Verification items for the finished model (mm, model axes). Round coordinates to 2 decimals unless told otherwise and drop trailing zeros. Write each loop counter-clockwise with the first axis right and the second up, starting at its lowest first coordinate (ties: lowest second). Pieces come first, ordered by that corner, then holes. Notation, with made-up numbers: (85, -6) - (109, -6) arc R15 ccw to (109, 9) - close; hole circle Ø10 at (73, 80). An arc over 180 degrees is marked (long way). Write each question's results on one line, items separated by ' | '.
```python
from build123d import *

# Parameters (mm, degrees)
SKETCH1_R           = 7
BOSS_EXTRUDE1_DEPTH = 0.5
SKETCH2_R           = 1.778
CUT_EXTRUDE2_DEPTH  = 1.5
SKETCH4_R           = 0.25
CUT_EXTRUDE3_DEPTH  = 1.5


with BuildPart() as part:
    # Sketch1 → Boss-Extrude1 (new body)
    with BuildSketch(Plane(origin=(0, 0, 0), x_dir=(1, 0, 0), z_dir=(0, 1, 0))):
        with BuildLine():
            Line((-6.25, 14.184057953), (-6.25, 11.399013115))
            ThreePointArc((-6.25, 11.399013115), (-9.192388155, 9.192388155), (-11.399013115, 6.25))
            Line((-11.399013115, 6.25), (-14.184057953, 6.25))
            ThreePointArc((-14.184057953, 6.25), (-15.5, 0), (-14.184057953, -6.25))
            Line((-14.184057953, -6.25), (-11.399013115, -6.25))
            ThreePointArc((-11.399013115, -6.25), (-9.192388155, -9.192388155), (-6.25, -11.399013115))
            Line((-6.25, -11.399013115), (-6.25, -14.184057953))
            ThreePointArc((-6.25, -14.184057953), (0, -15.5), (6.25, -14.184057953))
            Line((6.25, -14.184057953), (6.25, -11.399013115))
            ThreePointArc((6.25, -11.399013115), (9.192388155, -9.192388155), (11.399013115, -6.25))
            Line((11.399013115, -6.25), (14.184057953, -6.25))
            ThreePointArc((14.184057953, -6.25), (15.5, 0), (14.184057953, 6.25))
            Line((14.184057953, 6.25), (11.399013115, 6.25))
            ThreePointArc((11.399013115, 6.25), (9.192388155, 9.192388155), (6.25, 11.399013115))
            Line((6.25, 11.399013115), (6.25, 14.184057953))
            ThreePointArc((6.25, 14.184057953), (0, 15.5), (-6.25, 14.184057953))
        make_face()
        Circle(SKETCH1_R, mode=Mode.SUBTRACT)
    extrude(amount=BOSS_EXTRUDE1_DEPTH)

    # Sketch2 → Cut-Extrude2 (cut, through all)
    with BuildSketch(Plane(origin=(0, 0.5, 0), x_dir=(1, 0, 0), z_dir=(0, 1, 0))):
        with Locations((0, 13.3)):
            Circle(SKETCH2_R)
        with Locations((-2.381135215, 8.886517602)):
            Circle(SKETCH2_R)
        with Locations((-13.3, 0)):
            Circle(SKETCH2_R)
        with Locations((-8.886517602, 2.381135215)):
            Circle(SKETCH2_R)
        with Locations((-7.201882566, 7.201882566)):
            Circle(SKETCH2_R)
        with Locations((0, -13.3)):
            Circle(SKETCH2_R)
        with Locations((-2.381135215, -8.886517602)):
            Circle(SKETCH2_R)
        with Locations((-7.201882566, -7.201882566)):
            Circle(SKETCH2_R)
        with Locations((-8.886517602, -2.381135215)):
            Circle(SKETCH2_R)
        with Locations((2.381135215, 8.886517602)):
            Circle(SKETCH2_R)
        with Locations((7.201882566, 7.201882566)):
            Circle(SKETCH2_R)
        with Locations((8.886517602, 2.381135215)):
            Circle(SKETCH2_R)
        with Locations((13.3, 0)):
            Circle(SKETCH2_R)
        with Locations((8.886517602, -2.381135215)):
            Circle(SKETCH2_R)
        with Locations((7.201882566, -7.201882566)):
            Circle(SKETCH2_R)
        with Locations((2.381135215, -8.886517602)):
            Circle(SKETCH2_R)
    extrude(amount=-CUT_EXTRUDE2_DEPTH, mode=Mode.SUBTRACT)

    # Sketch4 → Cut-Extrude3 (cut, through all)
    with BuildSketch(Plane(origin=(0, 0.5, 0), x_dir=(1, 0, 0), z_dir=(0, 1, 0))):
        with Locations((-4, 13.25)):
            Circle(SKETCH4_R)
        with Locations((13.25, -4)):
            Circle(SKETCH4_R)
        with Locations((4, -13.25)):
            Circle(SKETCH4_R)
        with Locations((-4, -13.25)):
            Circle(SKETCH4_R)
        with Locations((4, 13.25)):
            Circle(SKETCH4_R)
    extrude(amount=-CUT_EXTRUDE3_DEPTH, mode=Mode.SUBTRACT)


solid = part.part
```
(1) Section check A-A (x = 0). Record the cut outline in (y, z).
Answer:
outline: (0, -15.5) - (0.5, -15.5) - (0.5, -15.08) - (0, -15.08) - close; (0, -11.52) - (0.5, -11.52) - (0.5, -7) - (0, -7) - close; (0, 7) - (0.5, 7) - (0.5, 11.52) - (0, 11.52) - close; (0, 15.08) - (0.5, 15.08) - (0.5, 15.5) - (0, 15.5) - close
(2) Thickness scan on L1, parallel to Z at x = -4, y = 0.2; L2, parallel to X at y = 0.2, z = -13.3; L3, parallel to Z at x = -0.5, y = 0.1. Record the ranges inside material, lowest first.
Answer:
L1: -14.97 to -13.5, -13 to -9.62, -8.15 to -5.74, 5.74 to 8.15, 9.62 to 13, 13.5 to 14.97 | L2: -6.25 to -4.24, -3.76 to -1.78, 1.78 to 3.76, 4.24 to 6.25 | L3: -15.49 to -15.01, -11.59 to -6.98, 6.98 to 11.59, 15.01 to 15.49
(3) Go/stop test with flat-tipped pins: pin 1 Ø3 at (x, z) = (-2.5, -6) entering from +Y; pin 2 Ø3 at (x, z) = (-2.38, -8.89) entering from +Y. Record where each tip stops, or that it passes through.
Answer:
pin 1: y = 0.5 | pin 2: through
(4) Section check B-B (z = 0). Record the cut outline in (x, y).
Answer:
outline: (-15.5, 0) - (-15.08, 0) - (-15.08, 0.5) - (-15.5, 0.5) - close; (-11.52, 0) - (-7, 0) - (-7, 0.5) - (-11.52, 0.5) - close; (7, 0) - (11.52, 0) - (11.52, 0.5) - (7, 0.5) - close; (15.08, 0) - (15.5, 0) - (15.5, 0.5) - (15.08, 0.5) - close
(5) Section check D-D (z = 12.5). Record the cut outline in (x, y).
Answer:
outline: (-6.25, 0) - (-1.59, 0) - (-1.59, 0.5) - (-6.25, 0.5) - close; (1.59, 0) - (6.25, 0) - (6.25, 0.5) - (1.59, 0.5) - close
(6) Section check C-C (x = -13.3). Record the cut outline in (y, z).
Answer:
outline: (0, -6.25) - (0.5, -6.25) - (0.5, -1.78) - (0, -1.78) - close; (0, 1.78) - (0.5, 1.78) - (0.5, 6.25) - (0, 6.25) - close
(7) Mould release check, pull along Z, two halves, no side actions. Record for faces 1 (the cylindrical face through (2.15, 0.25, -10.65)), 2 (the cylindrical face through (9.229, 0.246, -9.156)), 3 (the cylindrical face through (-7.43, 0.25, 5.44)), 4 (the cylindrical face through (-15.5, 0.2, -0.1)): released by +Z, released by -Z, zero draft, split by the parting line, or undercut.
Answer:
face 1: undercut | face 2: released by -Z | face 3: undercut | face 4: split by the parting line
